Part model, mm, in its own coordinate system. Face numbers are marked on the shaded views. Give positions to 0.01 mm unless a question says otherwise; leave off trailing zeros. Write each loop counter-clockwise with the first axis right and the second up, starting at its lowest first coordinate (ties: lowest second). Pieces come first, ordered by that corner, then holes.
Autodesk Inventor part; units mm, degrees
ref_plane "YZ Plane" through (0, 0, 0) normal (1, 0, 0) x (0, 1, 0)
ref_plane "XZ Plane" through (0, 0, 0) normal (0, 1, 0) x (-1, 0, 0)
ref_plane "XY Plane" through (0, 0, 0) normal (0, 0, 1) x (1, 0, 0)
sketch "Sketch1" plane through (0, 0, 0) normal (0, 0, 1) x (1, 0, 0)
  circle A0 centre (0, 0) radius 76.2
  circle A1 centre (0, 63.5) radius 3.3734
  circle A2 centre (0, 0) radius 38.1
  circle A3 centre (-31.75, 54.9926) radius 3.3734
  circle A4 centre (-54.9926, 31.75) radius 3.3734
  circle A5 centre (-63.5, 0) radius 3.3734
  circle A6 centre (-54.9926, -31.75) radius 3.3734
  circle A7 centre (-31.75, -54.9926) radius 3.3734
  circle A8 centre (0, -63.5) radius 3.3734
  circle A9 centre (31.75, -54.9926) radius 3.3734
  circle A10 centre (54.9926, -31.75) radius 3.3734
  circle A11 centre (63.5, 0) radius 3.3734
  circle A12 centre (54.9926, 31.75) radius 3.3734
  circle A13 centre (31.75, 54.9926) radius 3.3734
  dimension "d0" = 63.5
  dimension "d1" = 152.4
  dimension "d2" = 6.7469
  dimension "d3" = 76.2
  dimension "d6" = 360
extrude "Extrusion1" add sketch "Sketch1" along normal blind 6.35
sketch "Sketch2" plane through (0, 0, 6.35) normal (0, 0, 1) x (1, 0, 0)
  circle A0 centre (0, 0) radius 46.2375
  circle A1 centre (0, 0) radius 52.5875
  dimension "d10" = 92.475
  dimension "d11" = 6.35
extrude "Extrusion2" add sketch "Sketch2" along normal blind 12.7
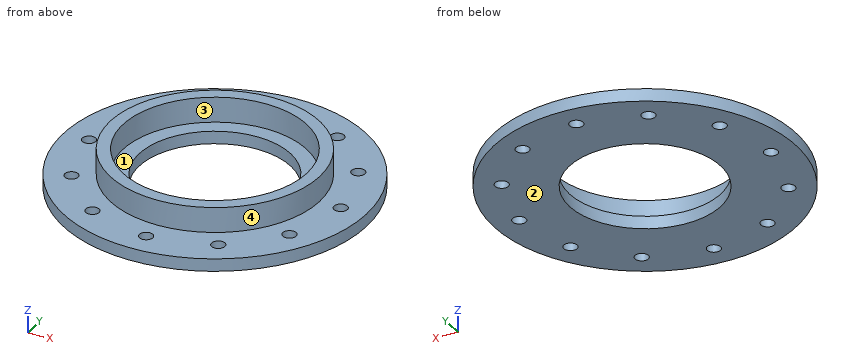
1) Saw through at B-B, the plane y = -22.5. Write the cut outline in (x, z), then the cut area to 3 significant figures.
Answers follow:
outline: (-72.8, 0) - (-30.75, 0) - (-30.75, 6.35) - (-40.39, 6.35) - (-40.39, 19.05) - (-47.53, 19.05) - (-47.53, 6.35) - (-72.8, 6.35) - close; (30.75, 0) - (72.8, 0) - (72.8, 6.35) - (47.53, 6.35) - (47.53, 19.05) - (40.39, 19.05) - (40.39, 6.35) - (30.75, 6.35) - close
area: 715 mm2
2) Saw through at C-C, the plane x = 14.5. Write the cut outline in (y, z), then the cut area to 3 significant figures.
Answers follow:
outline: (-74.81, 0) - (-35.23, 0) - (-35.23, 6.35) - (-43.91, 6.35) - (-43.91, 19.05) - (-50.55, 19.05) - (-50.55, 6.35) - (-74.81, 6.35) - close; (35.23, 0) - (74.81, 0) - (74.81, 6.35) - (50.55, 6.35) - (50.55, 19.05) - (43.91, 19.05) - (43.91, 6.35) - (35.23, 6.35) - close
area: 671 mm2
3) Wall check: L1, parallel to Y at x = 0, z = 4.5; L2, parallel to X at y = -55.5, z = 2.75; L3, parallel to Z at x = 26.5, y = 66.5. Give the ranges that are in metal, low to high.
Answers follow:
L1: y = -76.2 to -66.87, -60.13 to -38.1, 38.1 to 60.13, 66.87 to 76.2
L2: x = -52.21 to -35.09, -28.41 to 28.41, 35.09 to 52.21
L3: z = 0 to 6.35
4) Pin check, flat tips, straight feed: pin 1 Ø9 at (x, y) = (31.75, 54.99) entering from +Z; pin 2 Ø4 at (x, y) = (0, 63.5) entering from -Z; pin 3 Ø11 at (x, y) = (-31.75, 54.99) entering from -Z; pin 4 Ø8 at (y, z) = (13.5, 5.5) entering from +X. Stop position of each tip, or through.
Answers follow:
pin 1: stops at z = 6.35
pin 2: passes through
pin 3: stops at z = 0
pin 4: stops at x = 75.61
5) Saw through at A-A, the plane x = 32. Write the cut outline in (y, z).
Answers follow:
outline: (-69.16, 0) - (-58.36, 0) - (-58.36, 6.35) - (-69.16, 6.35) - close; (-51.63, 0) - (-20.68, 0) - (-20.68, 6.35) - (-33.38, 6.35) - (-33.38, 19.05) - (-41.73, 19.05) - (-41.73, 6.35) - (-51.63, 6.35) - close; (20.68, 0) - (51.63, 0) - (51.63, 6.35) - (41.73, 6.35) - (41.73, 19.05) - (33.38, 19.05) - (33.38, 6.35) - (20.68, 6.35) - close; (58.36, 0) - (69.16, 0) - (69.16, 6.35) - (58.36, 6.35) - close
6) Two-plate mould, pull along X, no slides. Class the marked faces 1, 2, 3 and 4: +X half, -X half, draft (parallel to the pull), parting line (faces both ways), or undercut.
Answers follow:
face 1: undercut
face 2: draft
face 3: undercut
face 4: parting line
7) Saw through at D-D, the plane z = 4.5. Count the separate pieces of the cut face and the enclosed holes in it, then the cut area to 3 significant figures.
Answers follow:
separate pieces: 1
enclosed holes: 13
area: 13,300 mm2
